Here's how the part is built. I have some questions about the finished solid (model axes, mm). A direction names the side the tool comes from. Round coordinates to 2 decimals unless told otherwise and drop trailing zeros. Write item = value, one per line. Start each with the question number.
(1) On a 3-axis mill with a long thin cutter (end or side, diameter ignored), from which of +Z, -Z, +X, -X, +Y, -Y can I reach the whole of each face in a straight line? I mean faces 4 (the flat face through (0, 190, 4.1)), 5 (the cylindrical face through (1.96, 98.73, 2.57)), 6 (the flat face through (0, 190, 0)). Say none if no direction works.
(2) If we mould it in two halves opening along X, with no side actions, what happens to faces 1 (the flat face through (0, 30, 3)), 2 (the cylindrical face through (-0.553, 286.714, 2.572)), 3 (the flat face through (2, 341, 1))? For each: released by +X, released by -X, zero draft, split by the parting line, or undercut.
(3) Will these pins go through, and if not, where does the flat tip stop? pin 1 Ø7 at (x, y) = (0, 223) entering from +Z; pin 2 Ø13.5 at (x, y) = (0, 342.5) entering from -Z; pin 3 Ø0.9 at (y, z) = (152.5, 8.5) entering from -X; pin 4 Ø7.5 at (x, y) = (-2, 165.5) entering from +Z.
(4) I need wall thicknesses on line 1 along Z through (x, y) = (-10.25, 262); line 2 along X through (y, z) = (157, 4); line 3 along X through (y, z) = (291, 6). Which ranges of each line are inside material? Lowest first, please.
```python
from build123d import *

# Parameters (mm, degrees)
BOSS_EXTRUDE1_DEPTH                              = 325
CBORE_FOR_M4_HEX_HEAD_MACHINE_SCREW1_D           = 4.5
CBORE_FOR_M4_HEX_HEAD_MACHINE_SCREW1_CBORE_D     = 8.5
CBORE_FOR_M4_HEX_HEAD_MACHINE_SCREW1_CBORE_DEPTH = 3.1
LPATTERN1_COUNT                                  = 6
LPATTERN1_PITCH                                  = 60


with BuildPart() as part:
    # Sketch1 → Boss-Extrude1 (new body)
    with BuildSketch(Plane.XZ.offset(-30)):
        with BuildLine():
            Line((-7.8, 1.5), (-10.8, 1.5))
            ThreePointArc((-10.8, 1.5), (-10.941421356, 1.441421356), (-11, 1.3))
            Line((-11, 1.3), (-11, 0))
            Line((-11, 0), (11, 0))
            Line((11, 0), (11, 1.3))
            ThreePointArc((11, 1.3), (10.941421356, 1.441421356), (10.8, 1.5))
            Line((10.8, 1.5), (7.8, 1.5))
            ThreePointArc((7.8, 1.5), (7.05, 2.249999999), (7.8, 2.999999999))
            Line((7.8, 2.999999999), (12.5, 2.999999999))
            ThreePointArc((12.5, 2.999999999), (13.207106782, 3.292893218), (13.5, 4))
            Line((13.5, 4), (13.5, 7.7))
            ThreePointArc((13.5, 7.7), (13.207106782, 8.407106781), (12.5, 8.7))
            Line((12.5, 8.7), (8.750000002, 8.7))
            Line((8.750000002, 8.7), (8.750000002, 7.599999996))
            Line((8.750000002, 7.599999996), (11.500000003, 7.599999996))
            ThreePointArc((11.500000003, 7.599999996), (11.853553391, 7.453553388), (11.999999999, 7.1))
            Line((11.999999999, 7.1), (11.999999999, 4.6))
            ThreePointArc((11.999999999, 4.6), (11.853553391, 4.246446612), (11.500000003, 4.100000003))
            Line((11.500000003, 4.100000003), (7.950000003, 4.100000003))
            ThreePointArc((7.950000003, 4.100000003), (7.750000003, 3.900000003), (7.550000003, 4.100000003))
            Line((7.550000003, 4.100000003), (-7.549999997, 4.100000003))
            ThreePointArc((-7.549999997, 4.100000003), (-7.749999997, 3.900000003), (-7.949999997, 4.100000003))
            Line((-7.949999997, 4.100000003), (-11.499999997, 4.100000003))
            ThreePointArc((-11.499999997, 4.100000003), (-11.853553386, 4.246446612), (-11.999999994, 4.6))
            Line((-11.999999994, 4.6), (-11.999999994, 7.1))
            ThreePointArc((-11.999999994, 7.1), (-11.853553386, 7.453553388), (-11.499999998, 7.599999996))
            Line((-11.499999998, 7.599999996), (-8.749999996, 7.599999996))
            Line((-8.749999996, 7.599999996), (-8.749999996, 8.7))
            Line((-8.749999996, 8.7), (-12.5, 8.7))
            ThreePointArc((-12.5, 8.7), (-13.207106782, 8.407106781), (-13.5, 7.7))
            Line((-13.5, 7.7), (-13.5, 4))
            ThreePointArc((-13.5, 4), (-13.207106782, 3.292893218), (-12.5, 2.999999999))
            Line((-12.5, 2.999999999), (-7.8, 2.999999999))
            ThreePointArc((-7.8, 2.999999999), (-7.05, 2.249999999), (-7.8, 1.5))
        make_face()
    extrude(amount=-BOSS_EXTRUDE1_DEPTH)

    # CBORE for M4 Hex Head Machine Screw1 (through all)
    with Locations(Plane.XY.offset(4.100000003)):
        with Locations((0, 42.5)):
            cbore_for_m4_hex_head_machine_screw1 = CounterBoreHole(CBORE_FOR_M4_HEX_HEAD_MACHINE_SCREW1_D / 2, CBORE_FOR_M4_HEX_HEAD_MACHINE_SCREW1_CBORE_D / 2, CBORE_FOR_M4_HEX_HEAD_MACHINE_SCREW1_CBORE_DEPTH)

    # LPattern1: CBORE for M4 Hex Head Machine Screw1 ×6
    with Locations(*[(0, i * LPATTERN1_PITCH, 0) for i in range(1, LPATTERN1_COUNT)]):
        add(cbore_for_m4_hex_head_machine_screw1, mode=Mode.SUBTRACT)


solid = part.part
```
Returned:
q1.face_4 = +Z, +Y, -Y
q1.face_5 = +Z
q1.face_6 = -Z, +X, -X, +Y, -Y
q2.face_1 = zero draft
q2.face_2 = undercut
q2.face_3 = undercut
q3.pin_1 = 1
q3.pin_2 = 0
q3.pin_3 = -13.44
q3.pin_4 = 4.1
q4.line_1 = 0 to 1.5, 3 to 4.1, 7.6 to 8.7
q4.line_2 = -13.5 to -7.92, -7.58 to 7.58, 7.92 to 13.5
q4.line_3 = -13.5 to -12, 12 to 13.5
